Autodesk Inventor part; units mm, degrees
ref_plane "YZ Plane" through (0, 0, 0) normal (1, 0, 0) x (0, 1, 0)
ref_plane "XZ Plane" through (0, 0, 0) normal (0, 1, 0) x (-1, 0, 0)
ref_plane "XY Plane" through (0, 0, 0) normal (0, 0, 1) x (1, 0, 0)
sketch "Sketch1" plane through (0, 0, 0) normal (0, 1, 0) x (-1, 0, 0)
  circle A0 centre (0, 0) radius 2.0828
  dimension "d4" = 4.1656
extrude "Body" add sketch "Sketch1" along normal blind 6.35
sketch "Sketch2" plane through (0, 0, 0) normal (1, 0, 0) x (0, 1, 0)
  line L0 (6.35, -2.0828) -> (6.35, 2.0828)
  line L1 (6.35, 0) -> (6.35, -4.3688)
  line L2 (8.0772, 0) -> (6.35, 0)
  line L3 (8.0772, 0) -> (8.0772, -4.1656)
  arc A0 (8.0772, -4.1656) -> (9.0169, 0) centre (-0.6859, 0) ccw
  line L4 (6.35, -4.3688) -> (8.0772, -4.1656)
  line L5 (8.0772, 0) -> (9.0169, 0)
  point P0 (0, 0)
  point P1 (6.35, -2.0828)
  dimension "d5" = 4.3688
  dimension "d13" = 1.7272
  dimension "d57" = 4.1656
  dimension "d58" = 9.7028
  dimension "d59" = 0
revolve "Head" add sketch "Sketch2" angle 360 about axis through (0, 8.0772, 0) along (0, -1, 0)
sketch "Sketch5" plane through (0, 0, 0) normal (1, 0, 0) x (0, 1, 0)
  line L0 (0, -2.0828) -> (6.35, -2.0828)
  line L1 (6.35, 4.3688) -> (6.35, -4.3688)
  line L2 (6.35, -2.0828) -> (6.35, 2.0828)
  line L3 (0.0745, -2.0828) -> (-0.2261, -2.6035)
  line L4 (-0.2261, -2.6035) -> (-0.3253, -2.6035)
  line L5 (-0.3253, -2.6035) -> (-0.626, -2.0828)
  line L6 (0.0686, -2.6035) -> (-0.7252, -2.6035) construction
  line L7 (-0.626, -2.0828) -> (0.0745, -2.0828)
  line L8 (0, -2.0828) -> (6.35, -2.0828)
  point P0 (0, 0)
  dimension "d31" = 30
  dimension "d32" = 60
  dimension "a" = 0.0992
  dimension "d46" = 0.7937
  dimension "d54" = 0.0686
  dimension "d55" = 0.5207
  dimension "d56" = 0.0992
feature "Thread" [suppressed]
sketch "Sketch6" plane through (0, 0, 0) normal (0, 0, 1) x (1, 0, 0)
  line L0 (0, 0) -> (-1.4859, 0)
  line L1 (2.0828, 0) -> (-2.0828, 0)
  line L2 (-1.4859, 0) -> (-2.4948, 1.0089)
  line L3 (-2.4948, 1.0089) -> (-2.9651, -1.2188)
  line L4 (-2.9651, -1.2188) -> (-1.4859, -1.2188)
  line L5 (-2.0828, 0) -> (-2.0828, 6.35)
  line L6 (-1.4859, -1.2188) -> (-1.4859, 0)
  line L7 (0, -2.7326) -> (0, 7.8638)
  point P0 (-2.0828, 0.5969)
  dimension "d49" = 1.4859
  dimension "d50" = 135
revolve "Tapered End" cut sketch "Sketch6" angle 360 about axis through (0, -10, 0) along (0, 1, 0)
sketch "Sketch7" plane through (0, 0, 0) normal (1, 0, 0) x (0, 1, 0)
  line L0 (6.35, 4.3688) -> (6.35, -4.3688)
  line L1 (7.6962, 0.6985) -> (7.6962, -0.6985)
  line L2 (7.6962, 0.6985) -> (9.7028, 0.6985)
  line L3 (9.7028, 0.6985) -> (9.7028, -0.6985)
  line L4 (9.7028, -0.6985) -> (7.6962, -0.6985)
  point P0 (0, 0)
  dimension "d61" = 1.397
  dimension "d62" = 0.6985
  dimension "d65" = 7.6962
  dimension "d66" = 2.0066
extrude "Flathead" cut sketch "Sketch7" against normal mid plane 12.7
equation "\"d56\" = a"
properties part number "Screw 8-32 Nylon 1.250" material "Black"
Verification items for the finished model (mm, model axes). A direction names the side the tool comes from. Coordinates: 2 decimals unless noted, no trailing zeros. Loops run counter-clockwise (first coordinate to the right, second up) from the corner with the lowest first, then second, coordinate; pieces in that order, holes last. Notation, with made-up numbers: M -40,25.5 L 14,25.5 A9 ccw 14,34.5 Z; hole C 57,-6 d5. An arc over 180 degrees is marked long. One line per item, written item: value.
1. Mould release check, pull along Z, two halves, no side actions. Record for faces 1 (the flat face through (0, 0, 0)), 2 (the flat face through (0, 8, 0.698)), 3 (the conical face through (-4.12, 7.59, 0.92)): pulls with the +Z half, pulls with the -Z half, needs draft (parallel to the pull), parting line crosses it, or undercut.
Answers follow:
face 1: needs draft
face 2: undercut
face 3: parting line crosses it
2. Material ranges on line 1 along Y through (x, z) = (-4, -0.5); line 2 along Z through (x, y) = (-2.5, 8); line 3 along X through (y, z) = (1, 0.5), recorded low to high. Write a range as from..to.
Answers follow:
line 1: 6.35..7.7
line 2: -3.34..-0.7, 0.7..3.34
line 3: -2.02..2.02
3. Gauge pin test, flat ends, axial feed: P1, Ø1, axis at x = -3.5, z = 2.5, coming from the +Y side; P2, Ø3, axis at y = 4.5, z = 1.5, coming from the -X side; P3, Ø5, axis at y = 3.5, z = 2.5, coming from the +X side. Record the tip position at first contact, or that the pin passes through.
Answers follow:
P1: y = 8.24
P2: x = -2.08
P3: x = 2.08
4. Section check B-B on y = 2.5. Record the cut outline in (x, z).
Answers follow:
outline: C 0,0 d4.17
5. Section check C-C on y = 6.5. Record the cut outline in (x, z).
Answers follow:
outline: C 0,0 d8.7
6. Section check A-A on z = 0. Record the cut outline in (x, y).
Answers follow:
outline: M -4.37,6.35 L -2.08,6.35 L -2.08,0.6 L -1.49,0 L 1.49,0 L 2.08,0.6 L 2.08,6.35 L 4.37,6.35 L 4.21,7.7 L -4.21,7.7 Z
7. Set-up check for faces 4 (the cylindrical face through (-1.987, 3.433, -0.626)), 5 (the flat face through (0, 7.696, 0)): record each of +Z, -Z, +X, -X, +Y, -Y from which the full face is reachable in a straight line by a thin tool's end or side.
Answers follow:
face 4: -Y
face 5: +X, -X, +Y
